Work out the finished part from the listing and answer in its coordinate system (mm). A direction names the side the tool comes from. Coordinates: 2 decimals unless noted, no trailing zeros. Order: outer loops, then holes, each group sorted by start corner. A loop starts at its lowest first (then second) coordinate and runs counter-clockwise, first axis right, second up. Notation, with made-up numbers: (-8, -12.5) - (10, -12.5) arc R12 ccw to (10, -6.5) - close; hole circle Ø8 at (88, 13.25). An arc over 180 degrees is marked (long way). Answer as a JSON object with one key per item and string values. Group by question number.
1) Section D-D (y = 22.5) is taken. Give the vertices of the cut face in (x, z) (3 decimals).
2) Section B-B (x = 12.7) is taken. Give the vertices of the cut face in (y, z) (3 decimals), plus the area to 3 significant figures.
3) A tool of negligible diameter and unlimited length cuts with its end or side. For faces 5 (the face through (14, 3.175, 81)), 6 (the face through (12.59, 1.57, 149.85)), from which of +Z, -Z, +X, -X, +Y, -Y can it reach the whole face along a straight path? Write none if from no direction.
4) Section A-A (z = 152.4) is taken. Give the vertices of the cut face in (x, y) (3 decimals).
5) Each of these flat-tipped pins is pushed along its axis until it touches: P1, Ø10, axis at x = 21.5, z = 101, coming from the +Y side (3 decimals); P2, Ø6.5, axis at y = 15.5, z = 94.5, coming from the +X side (3 decimals). Where does it stop, or does it pass through?
6) Section C-C (z = 64) is taken. Give the vertices of the cut face in (x, y) (3 decimals), plus the area to 3 significant figures.
7) The mould has two halves that part along Z. Classify faces 1 (the face through (1.565, 13.521, 143.615)), 2 (the face through (3.175, 14, 81)), 3 (the face through (7, 2, 165.1)), 4 (the face through (1.565, 15.265, 16.692)): released by +Z, released by -Z, zero draft, split by the parting line, or undercut.
8) Find the intervals of material crossed by line 1 along Z through (x, y) = (12.7, 0.7); line 2 along X through (y, z) = (1, 12.7); line 3 along X through (y, z) = (16.5, 74) (3 decimals), in increasing order.
Autodesk Inventor part; units mm, degrees
ref_plane "YZ Plane" through (0, 0, 0) normal (1, 0, 0) x (0, 1, 0)
ref_plane "XZ Plane" through (0, 0, 0) normal (0, 1, 0) x (-1, 0, 0)
ref_plane "XY Plane" through (0, 0, 0) normal (0, 0, 1) x (1, 0, 0)
sketch "Sketch1" plane through (0, 0, 0) normal (0, 0, 1) x (1, 0, 0)
  line L0 (0, 0) -> (3.175, 0)
  line L1 (3.175, 0) -> (3.175, 25.4)
  line L2 (3.175, 25.4) -> (0, 25.4)
  line L3 (0, 25.4) -> (0, 0)
  line L4 (0, 0) -> (25.4, 0)
  line L5 (25.4, 0) -> (25.4, 3.175)
  line L6 (25.4, 3.175) -> (0, 3.175)
  line L7 (0, 3.175) -> (0, 0)
  dimension "d0" = 3.175
  dimension "d1" = 25.4
extrude "Extrusion1" add sketch "Sketch1" along normal blind 165.1
sketch "Sketch2" plane through (3.175, 3.175, 0) normal (1, 0, 0) x (0, 0, -1)
  line L0 (-165.1, 0) -> (-165.1, 22.225)
  line L1 (0, -3.175) -> (-165.1, -3.175)
  point P0 (-146.05, 11.1125)
  point P1 (-19.05, 11.1125)
  dimension "d4" = 19.05
  dimension "d5" = 127
  dimension "d6" = 14.2875
hole "Hole1" at (3.175, 14.2875, 146.05) at (3.175, 14.2875, 19.05) direction (-1, 0, 0) diameter 5.1054 end through all
sketch "Sketch3" plane through (3.175, 3.175, 0) normal (0, 1, 0) x (1, 0, 0)
  line L0 (22.225, 0) -> (0, 0)
  line L1 (22.225, 0) -> (22.225, -165.1)
  line L2 (0, 0) -> (0, -165.1)
  point P0 (-3.175, 0)
  point P1 (9.525, -152.4)
  point P2 (9.525, -12.7)
  dimension "d14" = 12.7
  dimension "d15" = 139.7
  dimension "d16" = 12.7
  dimension "d17" = 9.525
hole "Hole2" at (12.7, 3.175, 152.4) at (12.7, 3.175, 12.7) direction (0, -1, 0) diameter 5.1054 end through all
properties part number "FRA_014_AngleBracketGearbox" material "Aluminum 6061"
Report:
{
 "1": {"outline": "(0, 0) - (3.175, 0) - (3.175, 165.1) - (0, 165.1) - close"},
 "2": {"outline": "(0, 0) - (3.175, 0) - (3.175, 10.147) - (0, 10.147) - close; (0, 15.253) - (3.175, 15.253) - (3.175, 149.847) - (0, 149.847) - close; (0, 154.953) - (3.175, 154.953) - (3.175, 165.1) - (0, 165.1) - close", "area": "492 mm²"},
 "3": {"face 5": "+Z, -Z, +X, +Y", "face 6": "+Y, -Y"},
 "4": {"outline": "(0, 0) - (10.147, 0) - (10.147, 3.175) - (3.175, 3.175) - (3.175, 25.4) - (0, 25.4) - close; (15.253, 0) - (25.4, 0) - (25.4, 3.175) - (15.253, 3.175) - close"},
 "5": {"P1": "stops at y = 3.175", "P2": "stops at x = 3.175"},
 "6": {"outline": "(0, 0) - (25.4, 0) - (25.4, 3.175) - (3.175, 3.175) - (3.175, 25.4) - (0, 25.4) - close", "area": "151 mm²"},
 "7": {"face 1": "undercut", "face 2": "zero draft", "face 3": "released by +Z", "face 4": "undercut"},
 "8": {"line 1": "z = 0 to 10.15, 15.25 to 149.85, 154.95 to 165.1", "line 2": "x = 0 to 10.15, 15.25 to 25.4", "line 3": "x = 0 to 3.175"}
}
